from build123d import *

# Parameters (mm, degrees)
BOSS_EXTRUDE1_DEPTH                 = 12.2
SKETCH2_R                           = 6.1
BOSS_EXTRUDE2_DEPTH                 = 5.8
BOSS_EXTRU_1_DEPTH                  = 5.8
ENL_V_MAT_EXTRU_1_DEPTH             = 30.050301203
SKETCH8_R                           = 0.75
BOSS_EXTRUDE5_DEPTH                 = 4
SKETCH3_R                           = 2.3
BOSS_EXTRUDE6_DEPTH                 = 4.5
DIAM_TRE_DU_PER_AGE_2_5_2_5_1_D     = 2.5
DIAM_TRE_DU_PER_AGE_2_5_2_5_1_DEPTH = 4
DIAM_TRE_DU_PER_AGE_2_5_2_5_1_TIP   = 0.751075774


with BuildPart() as part:
    # Sketch1 → Boss-Extrude1 (new body)
    with BuildSketch(Plane(origin=(0, 0, 0), x_dir=(0, 0, -1), z_dir=(1, 0, 0))):
        Polygon((-11.4, -11.25), (-11.4, 7.05), (-16.2, 7.05), (-16.2, 9.55), (-11.4, 9.55), (-11.4, 11.25), (11.4, 11.25), (11.4, 9.55), (16.2, 9.55), (16.2, 7.05), (11.4, 7.05), (11.4, -11.25), align=None)
    extrude(amount=BOSS_EXTRUDE1_DEPTH)

    # Sketch2 → Boss-Extrude2 (add)
    with BuildSketch(Plane(origin=(0, 11.25, 0), x_dir=(1, 0, 0), z_dir=(0, 1, 0))):
        with Locations(Location((6.1, -5.3, 0), (0, 0, 270))):
            Circle(SKETCH2_R)
    extrude(amount=BOSS_EXTRUDE2_DEPTH)

    # Sketch4 → Boss.-Extru.1 (add)
    with BuildSketch(Plane(origin=(0, 11.25, 0), x_dir=(1, 0, 0), z_dir=(0, 1, 0))):
        with BuildLine():
            Line((3.1, 0.5), (3.1, 0.01130869))
            ThreePointArc((3.1, 0.01130869), (6.1, 0.8), (9.1, 0.01130869))
            Line((9.1, 0.01130869), (9.1, 0.5))
            ThreePointArc((9.1, 0.5), (6.1, 3.5), (3.1, 0.5))
        make_face()
    extrude(amount=BOSS_EXTRU_1_DEPTH)

    # Sketch6 → Enlèv. mat.-Extru.1 (cut, through all)
    with BuildSketch(Plane(origin=(0, 9.55, 0), x_dir=(1, 0, 0), z_dir=(0, 1, 0))):
        with BuildLine():
            Line((5.525, -16.2), (6.675, -16.2))
            Line((6.675, -16.2), (6.675, -14.87856417))
            ThreePointArc((6.675, -14.87856417), (6.1, -12.95), (5.525, -14.87856417))
            Line((5.525, -14.87856417), (5.525, -16.2))
        make_face()
        with BuildLine():
            Line((5.525, 14.87856417), (5.525, 16.2))
            Line((5.525, 16.2), (6.675, 16.2))
            Line((6.675, 16.2), (6.675, 14.87856417))
            ThreePointArc((6.675, 14.87856417), (6.1, 12.95), (5.525, 14.87856417))
        make_face()
    extrude(amount=-ENL_V_MAT_EXTRU_1_DEPTH, mode=Mode.SUBTRACT)

    # Sketch8 → Boss-Extrude5 (add)
    with BuildSketch(Plane.XY.offset(11.4)):
        with Locations(Location((6.1, -6.25, 0), (0, 0, 180))):
            Circle(SKETCH8_R)
        with Locations(Location((7.7, -6.25, 0), (0, 0, 180))):
            Circle(SKETCH8_R)
        with Locations(Location((4.5, -6.25, 0), (0, 0, 180))):
            Circle(SKETCH8_R)
    extrude(amount=BOSS_EXTRUDE5_DEPTH)

    # Sketch3 → Boss-Extrude6 (add)
    with BuildSketch(Plane(origin=(0, 17.05, 0), x_dir=(1, 0, 0), z_dir=(0, 1, 0))):
        with Locations(Location((6.1, -5.3, 0), (0, 0, 270))):
            Circle(SKETCH3_R)
    extrude(amount=BOSS_EXTRUDE6_DEPTH)

    # Diamètre du perçage Ø2.5 (2.5)1
    with Locations(Plane(origin=(0, 21.55, 0), x_dir=(1, 0, 0), z_dir=(0, 1, 0))):
        with Locations((6.1, -5.3)):
            Hole(DIAM_TRE_DU_PER_AGE_2_5_2_5_1_D / 2, depth=DIAM_TRE_DU_PER_AGE_2_5_2_5_1_DEPTH)
            with Locations((0, 0, -(DIAM_TRE_DU_PER_AGE_2_5_2_5_1_DEPTH + DIAM_TRE_DU_PER_AGE_2_5_2_5_1_TIP / 2))):  # 118° drill point
                Cone(0, DIAM_TRE_DU_PER_AGE_2_5_2_5_1_D / 2, DIAM_TRE_DU_PER_AGE_2_5_2_5_1_TIP, mode=Mode.SUBTRACT)


solid = part.part
Source: CAD feature listing. Evaluate the final solid. Frame: model axes, mm. A direction names the side the tool comes from. Coordinates: 2 decimals unless noted, no trailing zeros. Loops run counter-clockwise (first coordinate to the right, second up) from the corner with the lowest first, then second, coordinate; pieces in that order, holes last. Notation, with made-up numbers: (18.25, -5.5) -> (28.25, -5.5) arc R22 cw to (28.25, 14.5) -> close; hole circle Ø10 at (31.5, 14). An arc over 180 degrees is marked (long way). Answer in a Markdown table with one row per item. Add a question column.
Q1. Section C-C on z = -14. Return the cut outline in (x, y).
Q2. Section B-B on y = -6.25. Return the cut outline in (x, z).
Q3. Pull-direction query (X, two-part tool) for faces 1 (the face through (5.525, 8, 16)), 2 (the face through (6, 17.05, 2)), 3 (the face through (6.2, 14.1, -3.5)); classes: pulls with the +X half, pulls with the -X half, needs draft (parallel to the pull), parting line crosses it, or undercut.
Q4. Section D-D on x = 10. Return the cut outline in (y, z).
Q5. Ray query, line 1 along X through (y, z) = (8, -14); line 2 along Y through (x, z) = (3.5, -1); line 3 along Z through (x, y) = (9.75, -4.5). Return the intervals inside material, ascending.
Q6. Reachability of faces 4 (the face through (6, 10, -11.4)), 5 (the face through (1, 11.25, 10)), 6 (the face through (8, -6, 15.4)), 7 (the face through (5.525, 8, -16)) from +Z, -Z, +X, -X, +Y, -Y: full face, straight path, thin tool, end or side. Return the list, or none.
Q7. Contact query for flat-ended pins moving along their axis: pin 1 Ø1.3 at (x, z) = (6.1, 14) entering from +Y; pin 2 Ø0.8 at (x, y) = (4, 10.5) entering from +Z; pin 3 Ø1.2 at (x, y) = (7.5, -6.5) entering from +Z. Output: stop coordinate, or through.
Q8. Section A-A on z = 14. Return the cut outline in (x, y), and give its area (3 significant figures).
Computed values:
| question | item | result |
|---|---|---|
| 1 | outline | (0, 7.05) -> (5.05, 7.05) -> (5.05, 9.55) -> (0, 9.55) -> close; (7.15, 7.05) -> (12.2, 7.05) -> (12.2, 9.55) -> (7.15, 9.55) -> close |
| 2 | outline | (0, -11.4) -> (12.2, -11.4) -> (12.2, 11.4) -> (8.45, 11.4) -> (8.45, 15.4) -> (6.95, 15.4) -> (6.95, 11.4) -> (6.85, 11.4) -> (6.85, 15.4) -> (5.35, 15.4) -> (5.35, 11.4) -> (5.25, 11.4) -> (5.25, 15.4) -> (3.75, 15.4) -> (3.75, 11.4) -> (0, 11.4) -> close |
| 3 | face 1 | undercut |
| 3 | face 2 | needs draft |
| 3 | face 3 | parting line crosses it |
| 4 | outline | (-11.25, -11.4) -> (7.05, -11.4) -> (7.05, -16.2) -> (9.55, -16.2) -> (9.55, -11.4) -> (11.25, -11.4) -> (11.25, 0.61) -> (17.05, 0.61) -> (17.05, 9.99) -> (11.25, 9.99) -> (11.25, 11.4) -> (9.55, 11.4) -> (9.55, 16.2) -> (7.05, 16.2) -> (7.05, 11.4) -> (-11.25, 11.4) -> close |
| 5 | line 1 | x = 0 to 5.05, 7.15 to 12.2 |
| 5 | line 2 | y = -11.25 to 17.05 |
| 5 | line 3 | z = -11.4 to 11.4 |
| 6 | face 4 | -Z, +X, -X, +Y |
| 6 | face 5 | +Z, -X, +Y |
| 6 | face 6 | +Z, +X, -X, -Y |
| 6 | face 7 | -Z, +Y, -Y |
| 7 | pin 1 | stops at y = -5.5 |
| 7 | pin 2 | stops at z = 11.4 |
| 7 | pin 3 | stops at z = 15.4 |
| 8 | outline | (0, 7.05) -> (5.05, 7.05) -> (5.05, 9.55) -> (0, 9.55) -> close; circle Ø1.5 at (4.5, -6.25); circle Ø1.5 at (6.1, -6.25); circle Ø1.5 at (7.7, -6.25); (7.15, 7.05) -> (12.2, 7.05) -> (12.2, 9.55) -> (7.15, 9.55) -> close |
| 8 | area | 30.6 mm^2 |
